Part model, mm, in its own coordinate system. Face numbers are marked on the shaded views. Coordinates: 2 decimals unless noted, no trailing zeros. Write each loop counter-clockwise with the first axis right and the second up, starting at its lowest first coordinate (ties: lowest second). Pieces come first, ordered by that corner, then holes. Notation, with made-up numbers: (10, 84) -> (45, 84) arc R17 cw to (45, 96) -> close; hole circle Ø7 at (64, -14). An arc over 180 degrees is marked (long way). Write item = value, one per line.
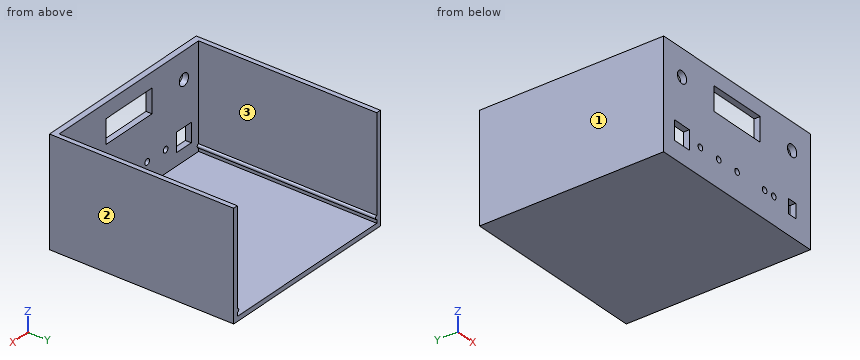
from build123d import *

# Parameters (mm, degrees)
F0_W     = 159
F0_H     = 90
F0_W_2   = 16
F0_H_2   = 16
F0_R     = 2.5
F0_W_3   = 8
F0_H_3   = 12
F0_R_2   = 5
F0_W_4   = 50
F0_H_4   = 20
F1_DEPTH = 5
F3_DEPTH = 150


with BuildPart() as f1:
    # F0 (on Front) → F1 (new body)
    with BuildSketch(Plane.XZ):
        with Locations((0, 45)):
            Rectangle(F0_W, F0_H)
        with Locations((-59.625, 22.5)):
            Rectangle(F0_W_2, F0_H_2, mode=Mode.SUBTRACT)
        with Locations((-39.75, 22.5)):
            Circle(F0_R, mode=Mode.SUBTRACT)
        with Locations((-19.875, 22.5)):
            Circle(F0_R, mode=Mode.SUBTRACT)
        with Locations((0, 22.5)):
            Circle(F0_R, mode=Mode.SUBTRACT)
        with Locations((29.8125, 22.5)):
            Circle(F0_R, mode=Mode.SUBTRACT)
        with Locations((39.75, 22.5)):
            Circle(F0_R, mode=Mode.SUBTRACT)
        with Locations((59.625, 22.5)):
            Rectangle(F0_W_3, F0_H_3, mode=Mode.SUBTRACT)
        with Locations((-59.625, 67.5)):
            Circle(F0_R_2, mode=Mode.SUBTRACT)
        with Locations((0, 67.5)):
            Rectangle(F0_W_4, F0_H_4, mode=Mode.SUBTRACT)
        with Locations((59.625, 67.5)):
            Circle(F0_R_2, mode=Mode.SUBTRACT)
    extrude(amount=F1_DEPTH)

    # F2 (on face) → F3 (join)
    with BuildSketch(Plane(origin=(0, 0, 0), x_dir=(-1, 0, 0), z_dir=(0, 1, 0))):
        with BuildLine():
            Line((75.5, 4), (-75.5, 4))
            Line((-75.5, 4), (-75.5, 7))
            ThreePointArc((-75.5, 7), (-74, 8.5), (-75.5, 10))
            Line((-75.5, 10), (-75.5, 90))
            Line((-75.5, 90), (-79.5, 90))
            Line((-79.5, 90), (-79.5, 0))
            Line((-79.5, 0), (79.5, 0))
            Line((79.5, 0), (79.5, 90))
            Line((79.5, 90), (75.5, 90))
            Line((75.5, 90), (75.5, 10))
            ThreePointArc((75.5, 10), (74, 8.5), (75.5, 7))
            Line((75.5, 7), (75.5, 4))
        make_face()
    extrude(amount=F3_DEPTH)


solid = f1.part
Q1. Pin check, flat tips, straight feed: pin 1 (6 mm diameter, centred on x = 0, z = 22.5, fed in from -Y); pin 2 (2 mm diameter, centred on x = 23, y = 106.5, fed in from +Z); pin 3 (3 mm diameter, centred on x = 30, z = 14.5, fed in from +Y); pin 4 (9 mm diameter, centred on x = -59.625, z = 67.5, fed in from -Y). Stop position of each tip, or through.
Model answer:
pin_1 = -5
pin_2 = 4
pin_3 = 0
pin_4 = through
Q2. Mould opens along X. For the marked faces 1, 2 and 3 say: released by +X, released by -X, zero draft, split by the parting line, or undercut.
Model answer:
face_1 = released by -X
face_2 = released by +X
face_3 = undercut
Q3. Saw through at B-B on y = 16.5. Give the cut face in (x, z).
Model answer:
outline = (-79.5, 0) -> (79.5, 0) -> (79.5, 90) -> (75.5, 90) -> (75.5, 10) arc R1.5 ccw to (75.5, 7) -> (75.5, 4) -> (-75.5, 4) -> (-75.5, 7) arc R1.5 ccw to (-75.5, 10) -> (-75.5, 90) -> (-79.5, 90) -> close
Q4. Saw through at A-A on z = 67.5. Give the cut face in (x, y) (3 decimals).
Model answer:
outline = (-79.5, -5) -> (-64.625, -5) -> (-64.625, 0) -> (-75.5, 0) -> (-75.5, 150) -> (-79.5, 150) -> close; (-54.625, -5) -> (-25, -5) -> (-25, 0) -> (-54.625, 0) -> close; (25, -5) -> (54.625, -5) -> (54.625, 0) -> (25, 0) -> close; (64.625, -5) -> (79.5, -5) -> (79.5, 150) -> (75.5, 150) -> (75.5, 0) -> (64.625, 0) -> close
Q5. Saw through at C-C on x = 39.75. Give the cut face in (y, z), and give its area (4 significant figures).
Model answer:
outline = (-5, 0) -> (150, 0) -> (150, 4) -> (0, 4) -> (0, 20) -> (-5, 20) -> close; (-5, 25) -> (0, 25) -> (0, 90) -> (-5, 90) -> close
area = 1,025 mm²
Q6. Saw through at D-D on x = 0. Give the cut face in (y, z), and give its area (3 significant figures).
Model answer:
outline = (-5, 0) -> (150, 0) -> (150, 4) -> (0, 4) -> (0, 20) -> (-5, 20) -> close; (-5, 25) -> (0, 25) -> (0, 57.5) -> (-5, 57.5) -> close; (-5, 77.5) -> (0, 77.5) -> (0, 90) -> (-5, 90) -> close
area = 925 mm²
Q7. Probe line 1 (X direction, y = 114.5, z = 81.5); line 2 (Z direction, x = 6, y = 16.5); line 3 (Z direction, x = 39.75, y = -2.15). List the from-to ranges inside material, lowest first. Write a range as from..to.
Model answer:
line_1 = -79.5..-75.5, 75.5..79.5
line_2 = 0..4
line_3 = 0..20, 25..90
